Autodesk Inventor part; units mm, degrees
ref_plane "YZ Plane" through (0, 0, 0) normal (1, 0, 0) x (0, 1, 0)
ref_plane "XZ Plane" through (0, 0, 0) normal (0, 1, 0) x (-1, 0, 0)
ref_plane "XY Plane" through (0, 0, 0) normal (0, 0, 1) x (1, 0, 0)
sketch "スケッチ1" plane through (0, 0, 0) normal (0, 0, 1) x (1, 0, 0)
  line L0 (7.5, 7.5) -> (-7.5, 7.5)
  line L1 (-7.5, 7.5) -> (-7.5, -7.5)
  line L2 (-7.5, -7.5) -> (7.5, -7.5)
  line L3 (7.5, -7.5) -> (7.5, 7.5)
  line L4 (7.5, 7.5) -> (-7.5, -7.5) construction
  line L5 (-7.5, 7.5) -> (7.5, -7.5) construction
  line L6 (-6, 6) -> (6, 6)
  line L7 (6, 6) -> (6, -6)
  line L8 (6, -6) -> (-6, -6)
  line L9 (-6, -6) -> (-6, 6)
  point P0 (0, 0)
  dimension "d0" = 15
  dimension "d1" = 15
  dimension "d2" = 1.5
extrude "押し出し1" add sketch "スケッチ1" along normal blind 550
sketch "スケッチ2" plane through (7.5, -7.5, 0) normal (1, 0, 0) x (0, 0, -1)
  circle A0 centre (-7, 7.5) radius 1.6
  circle A1 centre (-17, 7.5) radius 1.6
  line L0 (0, 0) -> (0, 15)
  circle A2 centre (-533, 7.5) radius 1.6
  circle A3 centre (-543, 7.5) radius 1.6
  line L1 (-550, 0) -> (-550, 15)
  point P0 (0, 7.5)
  point P1 (0, 7.5)
  dimension "d5" = 3.2
  dimension "d6" = 3.2
  dimension "d7" = 7
  dimension "d8" = 10
  dimension "d9" = 3.2
  dimension "d10" = 3.2
  dimension "d11" = 10
  dimension "d12" = 7
extrude "押し出し2" cut sketch "スケッチ2" against normal through all
properties part number "上昇機構_角柱4" material "アルミニウム 6061"
Geometry: final body of the model. Coordinates: model frame, mm. A direction names the side the tool comes from. Give positions to 0.01 mm unless a question says otherwise; leave off trailing zeros. Write each loop counter-clockwise with the first axis right and the second up, starting at its lowest first coordinate (ties: lowest second). Pieces come first, ordered by that corner, then holes.
(1) First-contact query: P1, Ø2.5, axis at y = 0, z = 17, coming from the -X side. Flat tip, straight axial feed; report the tip coordinate or a pass-through.
(2) Mould query, pull axis X, two halves, no side actions, for faces 1 (the flat face through (0, 6, 271)), 2 (the flat face through (0, 7.5, 271)), 3 (the flat face through (7.5, 0, 271)). Classes: released by +X, released by -X, zero draft, split by the parting line, or undercut.
(3) Access query for faces 4 (the flat face through (-7, 0, 550)), 5 (the flat face through (6, 0, 271)). Directions: +Z, -Z, +X, -X, +Y, -Y. A direction counts if a zero-diameter tool reaches every point of the face in a straight line with its end or side. Return the directions, or none.
(4) Cut plane A-A, the plane x = 3. Return loops of the section in (y, z), then the cut area to 3 significant figures.
(5) Cut plane B-B, the plane z = 490. Return loops of the section in (x, y).
(6) Ray query, line 1 (Y direction, x = -6.35, z = 17); line 2 (X direction, y = -4, z = 126). Return the intervals inside material, ascending.
Values follow:
1. P1: passes through
2. face 1: undercut
2. face 2: zero draft
2. face 3: released by +X
3. face 4: +Z, +X, -X, +Y, -Y
3. face 5: +Z, -Z
4. outline: (-7.5, 0) - (-6, 0) - (-6, 550) - (-7.5, 550) - close; (6, 0) - (7.5, 0) - (7.5, 550) - (6, 550) - close
4. area: 1,650 mm2
5. outline: (-7.5, -7.5) - (7.5, -7.5) - (7.5, 7.5) - (-7.5, 7.5) - close; hole (-6, -6) - (6, -6) - (6, 6) - (-6, 6) - close
6. line 1: y = -7.5 to -1.6, 1.6 to 7.5
6. line 2: x = -7.5 to -6, 6 to 7.5
